Could you check a few things on this model? Use its own coordinates, in mm. A direction names the side the tool comes from. Round coordinates to 2 decimals unless told otherwise and drop trailing zeros. Order: outer loops, then holes, each group sorted by start corner. A loop starts at its lowest first (then second) coordinate and runs counter-clockwise, first axis right, second up. Notation, with made-up numbers: (37.25, -6) -> (96.25, -6) arc R11 ccw to (96.25, -2) -> close; hole circle Ø9 at (37.25, 74.5). An arc over 180 degrees is marked (long way). One line per question, with ' | ' between items.
```python
from build123d import *

# Parameters (mm, degrees)
SKETCH_1_W               = 20
SKETCH_1_H               = 7.12
SKETCH_1_4_W             = 12
SKETCH_1_4_H             = 3
EXTRUDE_1_DEPTH          = 5
CUT_EXTRUDE_1_DEPTH      = 28.263289114
CUT_EXTRUDE_1_DEPTH_BACK = 28.263289114
SKETCH_3_R               = 1.5


with BuildPart() as part:
    # Sketch 1 → Revolve 1 (revolve)
    with BuildSketch(Plane.XY, mode=Mode.PRIVATE) as revolve_1_sk:
        with Locations((10, 3.56)):
            Rectangle(SKETCH_1_W, SKETCH_1_H)
    revolve(revolve_1_sk.sketch.rotate(Axis((-15.976954312, 0, 0), (1, 0, 0)), 90), axis=Axis((-15.976954312, 0, 0), (1, 0, 0)))

    # Sketch 1_4 → Cut-Revolve 1 (revolve, cut)
    with BuildSketch(Plane.XY, mode=Mode.PRIVATE) as cut_revolve_1_sk:
        with Locations((6, 1.5)):
            Rectangle(SKETCH_1_4_W, SKETCH_1_4_H)
    revolve(cut_revolve_1_sk.sketch.rotate(Axis((-15.976954312, 0, 0), (1, 0, 0)), 90), axis=Axis((-15.976954312, 0, 0), (1, 0, 0)), mode=Mode.SUBTRACT)

    # Sketch 2 → Extrude 1 (add)
    with BuildSketch(Plane(origin=(20, 0, 0), x_dir=(0, 0, -1), z_dir=(1, 0, 0))):
        Polygon((8.221467833, 0), (4.110733917, 7.12), (-4.110733917, 7.12), (-8.221467833, 0), (-4.110733917, -7.12), (4.110733917, -7.12), align=None)
    extrude(amount=EXTRUDE_1_DEPTH)

    # Sketch 3 → Cut-Extrude 1 (cut, two sides: drawn at the far end of the back side and taken through both)
    with BuildSketch(Plane(origin=(25, 0, 0), x_dir=(0, 0, -1), z_dir=(1, 0, 0)).offset(-CUT_EXTRUDE_1_DEPTH_BACK)):
        Circle(SKETCH_3_R)
    extrude(amount=CUT_EXTRUDE_1_DEPTH + CUT_EXTRUDE_1_DEPTH_BACK, mode=Mode.SUBTRACT)


solid = part.part
```
1. If we mould it in two halves opening along Y, with no side actions, what happens to faces 6 (the face through (6.08, -0.9, 2.86)), 7 (the face through (20, -6.4, -3.8)), 8 (the face through (22, 7.12, 0))? For each: pulls with the +Y half, pulls with the -Y half, needs draft (parallel to the pull), parting line crosses it, or undercut.
From the geometry:
face 6: undercut | face 7: needs draft | face 8: pulls with the +Y half
2. I need wall thicknesses on probe 1 along Y at (x, z) = (17.75, 0); probe 2 along Y at (x, z) = (9.25, 0); probe 3 along X at (y, z) = (-1.25, 1). Which ranges of each line are inside material? Lowest first, please.
From the geometry:
probe 1: y = -7.12 to -1.5, 1.5 to 7.12 | probe 2: y = -7.12 to -3, 3 to 7.12 | probe 3: x = 12 to 25
3. I want a section at C-C on x = 9.5. List the corners of the cut face in (y, z) for me.
From the geometry:
outline: circle Ø14.24 at (0, 0); hole circle Ø6 at (0, 0)
4. I'm going to push flat-ended pins straight in: pin 1 (1.8 mm diameter, centred on y = 5, z = 3.5, fed in from -X); pin 2 (3 mm diameter, centred on x = 22, y = 2, fed in from -Z); pin 3 (4 mm diameter, centred on x = 15, y = 3, fed in from -Z); pin 4 (8 mm diameter, centred on x = 12.5, z = 6.5, fed in from -Y). Where does each tip first touch, or does it pass through?
From the geometry:
pin 1: stops at x = 0 | pin 2: stops at z = -7.93 | pin 3: stops at z = -7.05 | pin 4: stops at y = -6.67
5. I want a section at D-D on z = -4.5. List the corners of the cut face in (x, y) for me.
From the geometry:
outline: (0, -5.52) -> (20, -5.52) -> (20, -6.45) -> (25, -6.45) -> (25, 6.45) -> (20, 6.45) -> (20, 5.52) -> (0, 5.52) -> close
6. I want a section at A-A on y = 0.75. List the corners of the cut face in (x, z) for me, and give its area (3 significant figures).
From the geometry:
outline: (0, -7.08) -> (20, -7.08) -> (20, -7.79) -> (25, -7.79) -> (25, -1.3) -> (12, -1.3) -> (12, -2.9) -> (0, -2.9) -> close; (0, 2.9) -> (12, 2.9) -> (12, 1.3) -> (25, 1.3) -> (25, 7.79) -> (20, 7.79) -> (20, 7.08) -> (0, 7.08) -> close | area: 258 mm²
7. On a 3-axis mill with a long thin cutter (end or side, diameter ignored), from which of +Z, -Z, +X, -X, +Y, -Y can I reach the whole of each face in a straight line? I mean faces 1 (the face through (20, -6.4, 3.6)), 2 (the face through (12, 1.3, -1.3)), 3 (the face through (20, 0, -7.4)), 4 (the face through (20, 6.4, -3.8)), 5 (the face through (20, 6.4, 3.6)). Say none if no direction works.
From the geometry:
face 1: +Z, -X, -Y | face 2: -X | face 3: -Z, -X | face 4: -Z, -X, +Y | face 5: +Z, -X, +Y
